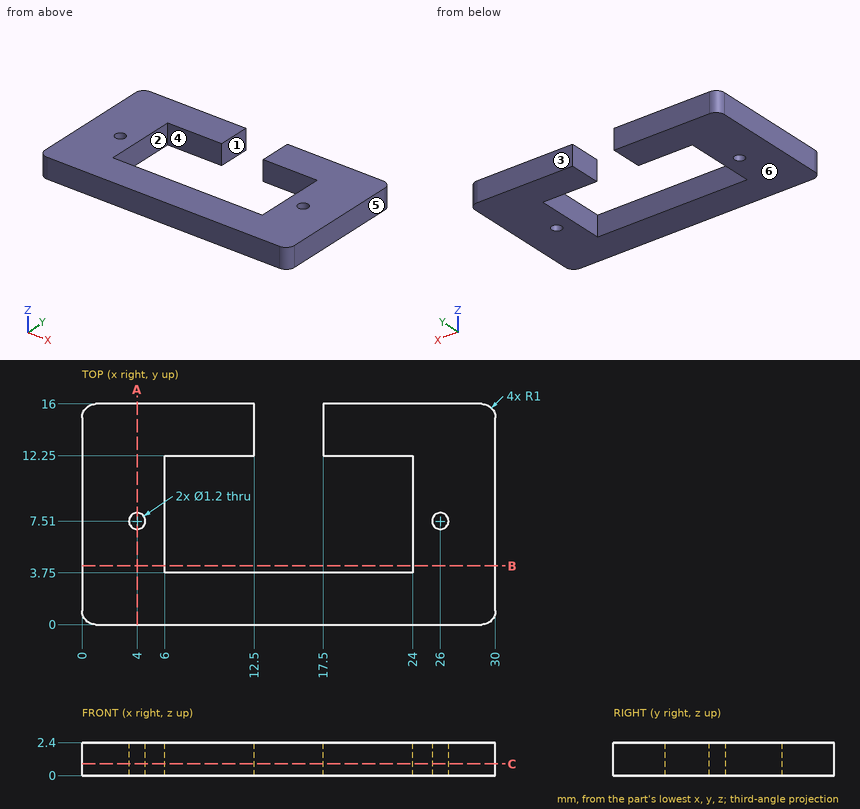
The figure shows three views and two pictorial views of one solid part (mm, origin at its lowest corner). Answer the questions. A direction names the side the tool comes from. Round coordinates to 2 decimals unless told otherwise and drop trailing zeros. Write each loop counter-clockwise with the first axis right and the second up, starting at its lowest first coordinate (ties: lowest second). Pieces come first, ordered by that corner, then holes. Notation, with made-up numbers: M 32.25,-28 L 85.25,-28 A7 cw 85.25,-20 Z; hole C 37.25,24.5 d4. An arc over 180 degrees is marked long. Write each question's results on one line, items separated by ' | '. Start each with the question number.
(1) The part is cut by section C-C, the plane z = 0.85. Write down the section's boundary in (x, y).
(2) This flat-tipped pin is pushed along its axis until it touches: P1, Ø1, axis at x = 4, y = 7.51, coming from the +Z side. Where does it stop, or does it pass through?
(3) The part is cut by section B-B, the plane y = 4.25. Write down the section's boundary in (x, z), and give its area (3 significant figures).
(4) Find the intervals of material crossed by line 1 (Y direction, x = 4, z = 1.4); line 2 (X direction, y = 9, z = 0.65); line 3 (Y direction, x = 18, z = 1.3), in increasing order.
(5) Determine the mould class of the marked faces 4, 5 and 6 for opening direction X: +X half, -X half, draft (parallel to the pull), parting line (faces both ways), or undercut.
(6) The part is cut by section A-A, the plane x = 4. Write down the section's boundary in (y, z).
(7) For the marked faces 1, 2 and 3, determine the directions among +Z, -Z, +X, -X, +Y, -Y from which every point of the face is accessible in a straight line to the end or side of a thin tool.
Worked answers:
1) outline: M 0,1 A1 ccw 1,0 L 29,0 A1 ccw 30,1 L 30,15 A1 ccw 29,16 L 17.5,16 L 17.5,12.25 L 24,12.25 L 24,3.75 L 6,3.75 L 6,12.25 L 12.5,12.25 L 12.5,16 L 1,16 A1 ccw 0,15 Z; hole C 4,7.51 d1.2; hole C 26,7.51 d1.2
2) P1: passes through
3) outline: M 0,0 L 6,0 L 6,2.4 L 0,2.4 Z; M 24,0 L 30,0 L 30,2.4 L 24,2.4 Z | area: 28.8 mm²
4) line 1: y = 0 to 6.91, 8.11 to 16 | line 2: x = 0 to 6, 24 to 30 | line 3: y = 0 to 3.75, 12.25 to 16
5) face 4: undercut | face 5: +X half | face 6: draft
6) outline: M 0,0 L 6.91,0 L 6.91,2.4 L 0,2.4 Z; M 8.11,0 L 16,0 L 16,2.4 L 8.11,2.4 Z
7) face 1: +Z, -Z, +Y | face 2: +Z, -Z | face 3: +Z, -Z, +X, -X, +Y
